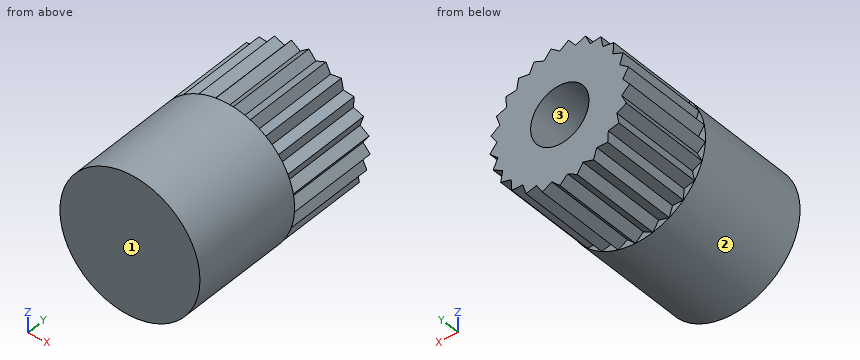
```python
from build123d import *

# Parameters (mm, degrees)
SKETCH_1_R           = 3
EXTRUDE_1_DEPTH      = 5
EXTRUDE_1_DEPTH_BACK = 4
SKETCH_2_OUTSIDE_W   = 10.474
SKETCH_2_OUTSIDE_H   = 10.474
CUT_EXTRUDE_1_DEPTH  = 4
SKETCH_3_R           = 1.25
CUT_EXTRUDE_2_DEPTH  = 7


with BuildPart() as part:
    # Эскиз1 → Бобышка-Вытянуть1 (new body, two sides)
    with BuildSketch(Plane(origin=(0, 0, 0), x_dir=(1, 0, 0), z_dir=(0, 1, 0))) as extrude_1_sk:
        Circle(SKETCH_1_R)
    extrude(amount=EXTRUDE_1_DEPTH)
    extrude(extrude_1_sk.sketch, amount=-EXTRUDE_1_DEPTH_BACK)

    # Эскиз2 outside → Вырез-Вытянуть1 (cut)
    with BuildSketch(Plane(origin=(0, 5, 0), x_dir=(1, 0, 0), z_dir=(0, 1, 0))):
        Rectangle(SKETCH_2_OUTSIDE_W, SKETCH_2_OUTSIDE_H)
        Polygon((0, 3), (0.338399731, 2.678709694), (0.746069661, 2.905749483), (0.993936292, 2.510396512), (1.445261022, 2.62892004), (1.587020181, 2.184345885), (2.053641318, 2.186905882), (2.080385755, 1.721044772), (2.532983777, 1.607480385), (2.443033042, 1.149604087), (2.853169549, 0.927050983), (2.652175577, 0.505929549), (2.994080185, 0.188371559), (2.694672167, -0.169534403), (2.946861752, -0.562143944), (2.567852594, -0.834345885), (2.714481157, -1.277337875), (2.279685399, -1.446732346), (2.311539728, -1.912271969), (1.848277186, -1.968215294), (1.763355757, -2.427050983), (1.30073492, -2.366028036), (1.104373658, -2.789329458), (0.671462695, -2.615174535), (0.375999701, -2.976344104), (0, -2.7), (-0.375999701, -2.976344104), (-0.671462695, -2.615174535), (-1.104373658, -2.789329458), (-1.30073492, -2.366028036), (-1.763355757, -2.427050983), (-1.848277186, -1.968215294), (-2.311539728, -1.912271969), (-2.279685399, -1.446732346), (-2.714481157, -1.277337875), (-2.567852594, -0.834345885), (-2.946861752, -0.562143944), (-2.694672167, -0.169534403), (-2.994080185, 0.188371559), (-2.652175577, 0.505929549), (-2.853169549, 0.927050983), (-2.443033042, 1.149604087), (-2.532983777, 1.607480385), (-2.080385755, 1.721044772), (-2.053641318, 2.186905882), (-1.587020181, 2.184345885), (-1.445261022, 2.62892004), (-0.993936292, 2.510396512), (-0.746069661, 2.905749483), (-0.338399731, 2.678709694), align=None, mode=Mode.SUBTRACT)
    extrude(amount=-CUT_EXTRUDE_1_DEPTH, mode=Mode.SUBTRACT)

    # Эскиз3 → Вырез-Вытянуть2 (cut)
    with BuildSketch(Plane(origin=(0, 5, 0), x_dir=(1, 0, 0), z_dir=(0, 1, 0))):
        Circle(SKETCH_3_R)
    extrude(amount=-CUT_EXTRUDE_2_DEPTH, mode=Mode.SUBTRACT)


solid = part.part
```
Here's how the part is built. I have some questions about the finished solid (model axes, mm). Face numbers are marked on the shaded views. Coordinates: 2 decimals unless noted, no trailing zeros. Write each loop counter-clockwise with the first axis right and the second up, starting at its lowest first coordinate (ties: lowest second). Pieces come first, ordered by that corner, then holes. Notation, with made-up numbers: (33, 65) -> (53, 65) arc R21 ccw to (53, 96) -> close; hole circle Ø4 at (-32, -20). An arc over 180 degrees is marked (long way). Use a Markdown table: item, result. Add a question column.
(1) If we section it at C-C, the plane z = 0.95: Write out the boundary of the cut face in (x, y).
(2) Please list where these lines run through material, in increasing order: line 1 (Z direction, x = 0, y = 0); line 2 (Y direction, x = 2.1, z = 2); line 3 (X direction, y = 3.75, z = -2.15).
(3) If we section it at D-D, the plane y = -2.75: Write out the boundary of the cut face in (x, z), and give its area (3 significant figures).
(4) If we section it at A-A, the plane z = 2.2: Write out the boundary of the cut face in (x, y).
(5) If we section it at B-B, the plane y = -0.5: Write out the boundary of the cut face in (x, z), and give its area (3 significant figures).
(6) We'd pull the mould along Z, two halves only. Please class the marked faces 1, 2 and 3: +Z half, -Z half, draft (parallel to the pull), parting line (faces both ways), or undercut.
(7) I'm going to push a flat-ended pin straight in: P1, Ø1.5, axis at y = 0.5, z = -2, coming from the +X side. Where does the tip first touch, or does it pass through?
Outcome:
| question | item | result |
|---|---|---|
| 1 | outline | (-2.85, -4) -> (2.85, -4) -> (2.85, 1) -> (2.61, 1) -> (2.61, 5) -> (0.81, 5) -> (0.81, -2) -> (-0.81, -2) -> (-0.81, 5) -> (-2.61, 5) -> (-2.61, 1) -> (-2.85, 1) -> close |
| 2 | line 1 | z = -3 to -1.25, 1.25 to 3 |
| 2 | line 2 | y = -4 to 1 |
| 2 | line 3 | x = -2.06 to 2.06 |
| 3 | outline | circle Ø6 at (0, 0) |
| 3 | area | 28.3 mm^2 |
| 4 | outline | (-2.04, -4) -> (2.04, -4) -> (2.04, 1) -> (1.81, 1) -> (1.81, 5) -> (-1.81, 5) -> (-1.81, 1) -> (-2.04, 1) -> close |
| 5 | outline | circle Ø6 at (0, 0); hole circle Ø2.5 at (0, 0) |
| 5 | area | 23.4 mm^2 |
| 6 | face 1 | draft |
| 6 | face 2 | parting line |
| 6 | face 3 | undercut |
| 7 | P1 | stops at x = 2.73 |
